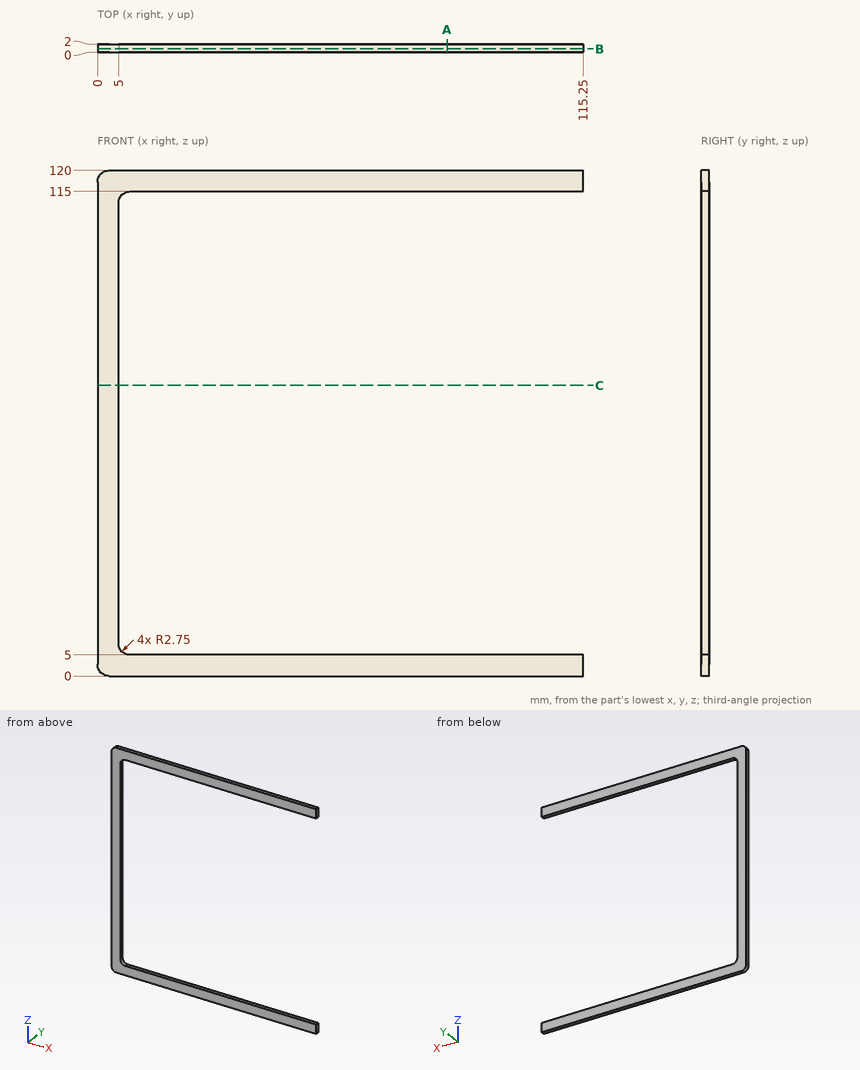
The drawing under review shows one solid part. Ordinate dimensions are in mm from its lowest x, y, z. Round coordinates to 2 decimals unless told otherwise and drop trailing zeros. Write each loop counter-clockwise with the first axis right and the second up, starting at its lowest first coordinate (ties: lowest second). Pieces come first, ordered by that corner, then holes. Notation, with made-up numbers: (-9.5, 11.25) -> (30.5, 11.25) arc R12 ccw to (30.5, 29.25) -> close; hole circle Ø10 at (38.5, 9). An arc over 180 degrees is marked (long way). One line per question, with ' | ' between items. Start each with the question number.
(1) For line 1 along Z through (x, y) = (25, 1.85); line 2 along X through (y, z) = (0.15, 45), list the stretches that pass through material, from the lowest coordinate up. Write a range as from..to.
(2) Add section C-C, the plane z = 69. Write out the cut boundary in (x, y).
(3) Add section B-B, the plane y = 0.85. Write out the cut boundary in (x, z).
(4) Add section A-A, the plane x = 83. Write out the cut boundary in (y, z), plus the area to 3 significant figures.
Answer list:
1) line 1: 0..5, 115..120 | line 2: 0..5
2) outline: (0, 0) -> (5, 0) -> (5, 2) -> (0, 2) -> close
3) outline: (0, 2.75) arc R2.75 ccw to (2.75, 0) -> (115.25, 0) -> (115.25, 5) -> (7.75, 5) arc R2.75 cw to (5, 7.75) -> (5, 112.25) arc R2.75 cw to (7.75, 115) -> (115.25, 115) -> (115.25, 120) -> (2.75, 120) arc R2.75 ccw to (0, 117.25) -> close
4) outline: (0, 0) -> (2, 0) -> (2, 5) -> (0, 5) -> close; (0, 115) -> (2, 115) -> (2, 120) -> (0, 120) -> close | area: 20.0 mm²
